Check sheet for the modelled part. Datum: model origin and axes. Units: mm. Face numbers are marked on the shaded views. A direction names the side the tool comes from. Round coordinates to 2 decimals unless told otherwise and drop trailing zeros. Write each loop counter-clockwise with the first axis right and the second up, starting at its lowest first coordinate (ties: lowest second). Pieces come first, ordered by that corner, then holes. Notation, with made-up numbers: (0.25, 21.5) -> (21.25, 21.5) arc R22 cw to (21.25, 50.5) -> close; hole circle Ø1 at (89, 49). An arc over 180 degrees is marked (long way). One line per item, written item: value.
from build123d import *

# Parameters (mm, degrees)
F1_DEPTH = 20
F2_W     = 10
F2_H     = 10
F3_DEPTH = 25
F4_W     = 4.138582
F4_H     = 10
F5_DEPTH = 25


with BuildPart() as f1:
    # F0 (on Front) → F1 (new body)
    with BuildSketch(Plane.XZ):
        Polygon((0, 20), (0, 0), (30, 0), (30, 5), align=None)
    extrude(amount=-F1_DEPTH)

    # F2 (on Right) → F3 (cut)
    with BuildSketch(Plane.YZ):
        with Locations((10, 15)):
            Rectangle(F2_W, F2_H)
    extrude(amount=F3_DEPTH, mode=Mode.SUBTRACT)

    # F4 (on Top) → F5 (cut)
    with BuildSketch(Plane.XY):
        with Locations((27.930709, 10)):
            Rectangle(F4_W, F4_H)
    extrude(amount=F5_DEPTH, mode=Mode.SUBTRACT)


solid = f1.part
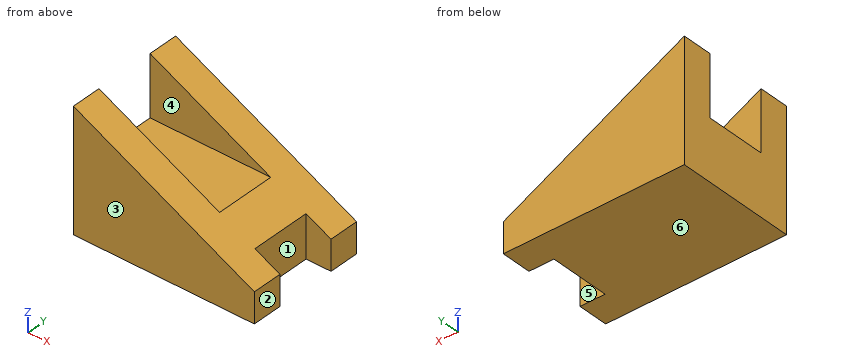
Item 1: Depth check by flat-ended pin: P1, Ø5, axis at y = 6.5, z = 11.5, coming from the +X side; P2, Ø5.5, axis at y = 10, z = 3.5, coming from the +X side; P3, Ø5, axis at x = 7, y = 8.5, coming from the +Z side. Enter the tip coordinate at first touch or a pass-through.
Answer:
P1: stops at x = 22
P2: stops at x = 25.86
P3: stops at z = 10
Item 2: Sectioned sample at B-B on z = 17.25. Enter the section's corners in (x, y).
Answer:
outline: (0, 0) -> (5.5, 0) -> (5.5, 5) -> (0, 5) -> close; (0, 15) -> (5.5, 15) -> (5.5, 20) -> (0, 20) -> close
Item 3: Sectioned sample at A-A on x = 28.5. Enter the section's corners in (y, z), and give its area (3 significant figures).
Answer:
outline: (0, 0) -> (5, 0) -> (5, 5.75) -> (0, 5.75) -> close; (15, 0) -> (20, 0) -> (20, 5.75) -> (15, 5.75) -> close
area: 57.5 mm^2
Item 4: Sectioned sample at D-D on y = 14.25. Enter the section's corners in (x, z), and give its area (3 significant figures).
Answer:
outline: (0, 0) -> (25.86, 0) -> (25.86, 7.07) -> (20, 10) -> (0, 10) -> close
area: 250 mm^2
Item 5: Mould release check, pull along Y, two halves, no side actions. Record for the marked faces 1, 2 and 3: pulls with the +Y half, pulls with the -Y half, needs draft (parallel to the pull), parting line crosses it, or undercut.
Answer:
face 1: undercut
face 2: needs draft
face 3: pulls with the -Y half
Item 6: Sectioned sample at C-C on z = 3.5. Enter the section's corners in (x, y).
Answer:
outline: (0, 0) -> (30, 0) -> (30, 5) -> (25.86, 5) -> (25.86, 15) -> (30, 15) -> (30, 20) -> (0, 20) -> close
Item 7: Thickness scan on line 1 (Y direction, x = 7, z = 13); line 2 (X direction, y = 10.75, z = 5.5); line 3 (Z direction, x = 7.5, y = 10). Record the ranges inside material, lowest first.
Answer:
line 1: y = 0 to 5, 15 to 20
line 2: x = 0 to 25.86
line 3: z = 0 to 10
Item 8: Tool access check on the marked faces 4, 5 and 6. Record the directions out of +Z, -Z, +X, -X, +Y, -Y that give a thin tool (end or side, any length) a straight path to the whole face; none if there is none.
Answer:
face 4: +Z, +X, -X
face 5: +Z, -Z, +X
face 6: -Z, +X, -X, +Y, -Y
